Build history of the part. All positions in model axes, mm. Face numbers are marked on the shaded views. Round coordinates to 2 decimals unless told otherwise and drop trailing zeros. Write each loop counter-clockwise with the first axis right and the second up, starting at its lowest first coordinate (ties: lowest second). Pieces come first, ordered by that corner, then holes. Notation, with made-up numbers: (71, 30) - (79, 30) arc R27 cw to (79, 61) - close; hole circle Ø11 at (31, 44.5). An arc over 180 degrees is marked (long way). One line per question, with ' | ' between items.
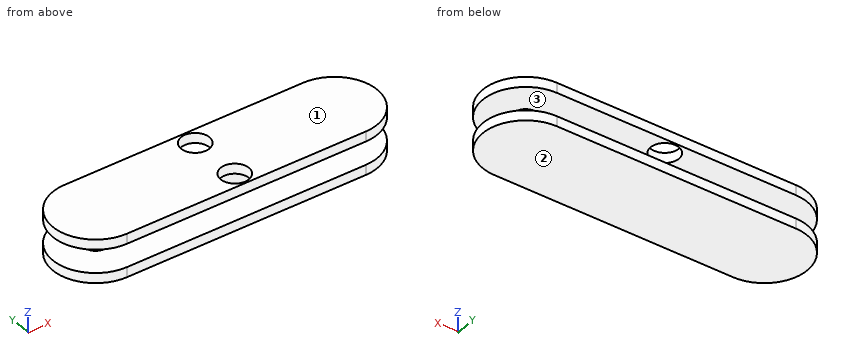
from build123d import *

# Parameters (mm, degrees)
F0_W          = 97.9224070907
F0_H          = 9.2892860994
F1_DEPTH      = 13.716
F1_DEPTH_BACK = 3.81
F0_H_2        = 12.6795382239
F2_DEPTH      = 0.254
F2_DEPTH_BACK = 3.81
F3_START      = 9.398
F3_DEPTH      = 4.064
F4_R          = 5.715
F5_DEPTH      = 4.572


with BuildPart() as f1:
    # F0 (on Top) → F1 (new body, two sides)
    with BuildSketch(Plane.XY) as f1_sk:
        Rectangle(F0_W, F0_H)
        with BuildLine():
            ThreePointArc((48.9612035453, -4.6446430497), (53.605846595, 0), (48.9612035453, 4.6446430497))
            Line((48.9612035453, 4.6446430497), (48.9612035453, -4.6446430497))
        make_face()
        with BuildLine():
            Line((-48.9612035453, -4.6446430497), (-48.9612035453, 4.6446430497))
            ThreePointArc((-48.9612035453, 4.6446430497), (-53.605846595, 0), (-48.9612035453, -4.6446430497))
        make_face()
    extrude(amount=F1_DEPTH)
    extrude(f1_sk.sketch, amount=-F1_DEPTH_BACK)

    # F0 (on Top) → F2 (join, two sides)
    with BuildSketch(Plane.XY) as f2_sk:
        with Locations((0, -10.9844121616)):
            Rectangle(F0_W, F0_H_2)
        with BuildLine():
            Line((-48.9612035453, 4.6446430497), (-48.9612035453, 17.3241812736))
            ThreePointArc((-48.9612035453, 17.3241812736), (-66.2853848189, 0), (-48.9612035453, -17.3241812736))
            Line((-48.9612035453, -17.3241812736), (-48.9612035453, -4.6446430497))
            ThreePointArc((-48.9612035453, -4.6446430497), (-53.605846595, 0), (-48.9612035453, 4.6446430497))
        make_face()
        with Locations((0, 10.9844121616)):
            Rectangle(F0_W, F0_H_2)
        with BuildLine():
            ThreePointArc((48.9612035453, -17.3241812736), (66.2853848189, 0), (48.9612035453, 17.3241812736))
            Line((48.9612035453, 17.3241812736), (48.9612035453, 4.6446430497))
            ThreePointArc((48.9612035453, 4.6446430497), (53.605846595, 0), (48.9612035453, -4.6446430497))
            Line((48.9612035453, -4.6446430497), (48.9612035453, -17.3241812736))
        make_face()
    extrude(amount=F2_DEPTH)
    extrude(f2_sk.sketch, amount=-F2_DEPTH_BACK)

    # F2_face (on face) → F3 (join)
    with BuildSketch(Plane.XY.offset(0.254).offset(F3_START)):
        with BuildLine():
            Line((-48.9612035453, -17.3241812736), (48.9612035453, -17.3241812736))
            ThreePointArc((48.9612035453, -17.3241812736), (66.2853848189, 0), (48.9612035453, 17.3241812736))
            Line((48.9612035453, 17.3241812736), (-48.9612035453, 17.3241812736))
            ThreePointArc((-48.9612035453, 17.3241812736), (-66.2853848189, 0), (-48.9612035453, -17.3241812736))
        make_face()
        with BuildLine():
            Line((48.9612035453, -4.6446430497), (-48.9612035453, -4.6446430497))
            ThreePointArc((-48.9612035453, -4.6446430497), (-53.605846595, 0), (-48.9612035453, 4.6446430497))
            Line((-48.9612035453, 4.6446430497), (48.9612035453, 4.6446430497))
            ThreePointArc((48.9612035453, 4.6446430497), (53.605846595, 0), (48.9612035453, -4.6446430497))
        make_face(mode=Mode.SUBTRACT)
    extrude(amount=F3_DEPTH)

    # F4 (on face) → F5 (cut)
    with BuildSketch(Plane.XY.offset(13.716)):
        with Locations((0, 10.922)):
            Circle(F4_R)
        with Locations((0, -10.922)):
            Circle(F4_R)
    extrude(amount=-F5_DEPTH, mode=Mode.SUBTRACT)


solid = f1.part
Q1. Drop flat-ended pins along their axis: pin 1 (6 mm diameter, centred on y = 12.5, z = 0, fed in from -X); pin 2 (1 mm diameter, centred on x = 47, z = 7.5, fed in from -Y); pin 3 (3 mm diameter, centred on y = -4.5, z = 4, fed in from +X). Give the stop position or say it passes through.
Found:
pin 1: x = -63.45 | pin 2: y = -4.64 | pin 3: x = 52.51
Q2. Pull direction Z, two halves, no side cores. Call the marked faces 1, 2 and 3: +Z half, -Z half, draft (parallel to the pull), parting line (faces both ways), or undercut.
Found:
face 1: +Z half | face 2: -Z half | face 3: undercut
Q3. Saw through at A-A, the plane x = 0. List the corners of the cut face in (y, z).
Found:
outline: (-17.32, -3.81) - (17.32, -3.81) - (17.32, 0.25) - (4.64, 0.25) - (4.64, 9.65) - (5.21, 9.65) - (5.21, 13.72) - (-5.21, 13.72) - (-5.21, 9.65) - (-4.64, 9.65) - (-4.64, 0.25) - (-17.32, 0.25) - close; (-17.32, 9.65) - (-16.64, 9.65) - (-16.64, 13.72) - (-17.32, 13.72) - close; (16.64, 9.65) - (17.32, 9.65) - (17.32, 13.72) - (16.64, 13.72) - close
Q4. Drill centre lines: L1, parallel to Y at x = 0, z = 12.85; L2, parallel to Z at x = -38, y = -12; L3, parallel to Y at x = -23, z = 2.5. Where is each one in solid material? Low to high. Write a range as from..to.
Found:
L1: -17.32..-16.64, -5.21..5.21, 16.64..17.32 | L2: -3.81..0.25, 9.65..13.72 | L3: -4.64..4.64
Q5. Saw through at B-B, the plane y = 0. List the corners of the cut face in (x, z), then the cut area to 3 significant figures.
Found:
outline: (-66.29, -3.81) - (66.29, -3.81) - (66.29, 0.25) - (53.61, 0.25) - (53.61, 9.65) - (66.29, 9.65) - (66.29, 13.72) - (-66.29, 13.72) - (-66.29, 9.65) - (-53.61, 9.65) - (-53.61, 0.25) - (-66.29, 0.25) - close | area: 2,090 mm^2
Q6. Saw through at C-C, the plane x = -39. List the corners of the cut face in (y, z).
Found:
outline: (-17.32, -3.81) - (17.32, -3.81) - (17.32, 0.25) - (4.64, 0.25) - (4.64, 9.65) - (17.32, 9.65) - (17.32, 13.72) - (-17.32, 13.72) - (-17.32, 9.65) - (-4.64, 9.65) - (-4.64, 0.25) - (-17.32, 0.25) - close
Q7. Saw through at D-D, the plane y = 14.5. List the corners of the cut face in (x, z).
Found:
outline: (-58.44, -3.81) - (58.44, -3.81) - (58.44, 0.25) - (-58.44, 0.25) - close; (-58.44, 9.65) - (-4.46, 9.65) - (-4.46, 13.72) - (-58.44, 13.72) - close; (4.46, 9.65) - (58.44, 9.65) - (58.44, 13.72) - (4.46, 13.72) - close
